For this review, take the finished solid that the model builds, in its own axes (mm). A direction names the side the tool comes from. Give positions to 0.01 mm unless a question says otherwise; leave off trailing zeros. Order: outer loops, then holes, each group sorted by start corner. A loop starts at its lowest first (then second) coordinate and runs counter-clockwise, first axis right, second up.
from build123d import *

# Parameters (mm, degrees)
AUFSATZ_LINEAR_AUSTRAGEN1_DEPTH = 3
AUFSATZ_LINEAR_AUSTRAGEN3_DEPTH = 3
AUFSATZ_LINEAR_AUSTRAGEN2_DEPTH = 20
AUFSATZ_LINEAR_AUSTRAGEN4_DEPTH = 8
FASE1_SIZE                      = 8
SCHNITT_LINEAR_AUSTRAGEN1_REACH = 119.702
SKIZZE5_R                       = 2.6
SCHNITT_LINEAR_AUSTRAGEN2_REACH = 178.395
SKIZZE6_R                       = 2.6
SCHNITT_LINEAR_AUSTRAGEN3_REACH = 178.395
SKIZZE7_R                       = 2.6
SCHNITT_LINEAR_AUSTRAGEN4_REACH = 140.701
SKIZZE8_R                       = 2.6


with BuildPart() as part:
    # Skizze1 → Aufsatz-Linear austragen1 (new body)
    with BuildSketch(Plane(origin=(0, 0, 0), x_dir=(1, 0, 0), z_dir=(0, 1, 0))):
        Polygon((-10, -84.737699009), (10, -84.737699009), (10, -64.737699009), (61.064491924, 23.708595467), (78.385, 33.708595467), (68.385, 51.029103542), (51.064491924, 41.029103542), (-51.064491924, 41.029103542), (-68.385, 51.029103542), (-78.385, 33.708595467), (-61.064491924, 23.708595467), (-10, -64.737699009), align=None)
    extrude(amount=AUFSATZ_LINEAR_AUSTRAGEN1_DEPTH)

    # Skizze3 → Aufsatz-Linear austragen3 (add)
    with BuildSketch(Plane.XZ):
        Polygon((0, -51.029103542), (-10, -41.029103542), (10, -41.029103542), align=None)
    extrude(amount=-AUFSATZ_LINEAR_AUSTRAGEN3_DEPTH)

    # Skizze2 → Aufsatz-Linear austragen2 (add)
    with BuildSketch(Plane.XZ):
        Polygon((-10.057735027, 64.637699009), (10.057735027, 64.637699009), (11.789785834, 61.637699009), (-11.789785834, 61.637699009), align=None)
        Polygon((61.006756897, -23.608595467), (50.94902187, -41.029103542), (47.484920255, -41.029103542), (59.27470609, -20.608595467), align=None)
        Polygon((-50.94902187, -41.029103542), (-61.006756897, -23.608595467), (-59.27470609, -20.608595467), (-47.484920255, -41.029103542), align=None)
    extrude(amount=AUFSATZ_LINEAR_AUSTRAGEN2_DEPTH)

    # Skizze4 → Aufsatz-Linear austragen4 (add)
    with BuildSketch(Plane.XZ):
        Polygon((-11.789785834, 61.637699009), (-16.408587988, 53.637699009), (-13.408587988, 53.637699009), (-8.789785834, 61.637699009), align=None)
        Polygon((11.789785834, 61.637699009), (8.789785834, 61.637699009), (13.408587988, 53.637699009), (16.408587988, 53.637699009), align=None)
        Polygon((59.27470609, -20.608595467), (54.655903936, -12.608595467), (53.155903936, -15.206671678), (57.77470609, -23.206671678), align=None)
        Polygon((47.484920255, -41.029103542), (48.984920255, -38.431027331), (39.747315948, -38.431027331), (38.247315948, -41.029103542), align=None)
        Polygon((-47.484920255, -41.029103542), (-38.247315948, -41.029103542), (-39.747315948, -38.431027331), (-48.984920255, -38.431027331), align=None)
        Polygon((-59.27470609, -20.608595467), (-57.77470609, -23.206671678), (-53.155903936, -15.206671678), (-54.655903936, -12.608595467), align=None)
    extrude(amount=AUFSATZ_LINEAR_AUSTRAGEN4_DEPTH)

    # Fase1
    # the kernel refuses this chamfer: 8 mm, written as the material it takes off along each edge
    with BuildSketch(Plane(origin=(-42.869171984, -8, -33.023814062), x_dir=(0.023812127644089447, 0.9996219169112968, 0.013747938305292782), z_dir=(-0.5000000000000003, 0, 0.8660254037844386))) as fase1_piece_1_section:
        Polygon((FASE1_SIZE * 0.999621916911, FASE1_SIZE * 0.0274958766106), (-FASE1_SIZE * 0.0274958766106, FASE1_SIZE * 0.999621916911), (0, 0), align=None)
    fase1_piece_1 = extrude(amount=44.146927807, mode=Mode.PRIVATE)
    fase1_piece_1 = split(fase1_piece_1, bisect_by=Plane(origin=(-56.186972779, 0, -15.224609283), z_dir=(0, -1, 0)), keep=Keep.TOP, mode=Mode.PRIVATE)
    add(fase1_piece_1, mode=Mode.SUBTRACT)
    with BuildSketch(Plane(origin=(-27.960583996, -8, -58.846245927), x_dir=(0.02381212764409005, 0.9996219169112968, 0.013747938305293118), z_dir=(-0.5, 0, 0.8660254037844387))) as fase1_piece_2_section:
        Polygon((FASE1_SIZE * 0.999621916911, FASE1_SIZE * 0.0274958766106), (-FASE1_SIZE * 0.0274958766106, FASE1_SIZE * 0.999621916911), (0, 0), align=None)
    fase1_piece_2 = extrude(amount=44.146927807, mode=Mode.PRIVATE)
    fase1_piece_2 = split(fase1_piece_2, bisect_by=Plane(origin=(-41.278384791, 0, -41.047041147), z_dir=(0, -1, 0)), keep=Keep.TOP, mode=Mode.PRIVATE)
    add(fase1_piece_2, mode=Mode.SUBTRACT)
    with BuildSketch(Plane(origin=(50.0340479, -8, -20.613884946), x_dir=(-0.023812127644090117, 0.9996219169112968, 0.013747938305293118), z_dir=(-0.49999999999999895, 0, -0.8660254037844393))) as fase1_piece_3_section:
        Polygon((FASE1_SIZE * 0.999621916911, FASE1_SIZE * 0.0274958766106), (-FASE1_SIZE * 0.0274958766106, FASE1_SIZE * 0.999621916911), (0, 0), align=None)
    fase1_piece_3 = extrude(amount=44.146927807, mode=Mode.PRIVATE)
    fase1_piece_3 = split(fase1_piece_3, bisect_by=Plane(origin=(41.278384791, 0, -41.047041147), z_dir=(0, -1, 0)), keep=Keep.TOP, mode=Mode.PRIVATE)
    add(fase1_piece_3, mode=Mode.SUBTRACT)
    with BuildSketch(Plane(origin=(64.942635888, -8, 5.208546918), x_dir=(-0.023812127644090537, 0.9996219169112968, 0.013747938305293455), z_dir=(-0.5000000000000016, 0, -0.8660254037844378))) as fase1_piece_4_section:
        Polygon((FASE1_SIZE * 0.999621916911, FASE1_SIZE * 0.0274958766106), (-FASE1_SIZE * 0.0274958766106, FASE1_SIZE * 0.999621916911), (0, 0), align=None)
    fase1_piece_4 = extrude(amount=44.146927807, mode=Mode.PRIVATE)
    fase1_piece_4 = split(fase1_piece_4, bisect_by=Plane(origin=(56.186972779, 0, -15.224609283), z_dir=(0, -1, 0)), keep=Keep.TOP, mode=Mode.PRIVATE)
    add(fase1_piece_4, mode=Mode.SUBTRACT)
    with BuildSketch(Plane(origin=(-7.164875916, -8, 53.637699009), x_dir=(0, -0.02749587661058627, 0.9996219169112968), z_dir=(1, 0, 0))) as fase1_piece_5_section:
        Polygon((FASE1_SIZE * 0.999621916911, -FASE1_SIZE * 0.0274958766106), (-FASE1_SIZE * 0.0274958766106, -FASE1_SIZE * 0.999621916911), (0, 0), align=None)
    fase1_piece_5 = extrude(amount=44.146927807, mode=Mode.PRIVATE)
    fase1_piece_5 = split(fase1_piece_5, bisect_by=Plane(origin=(14.908587988, 0, 61.735979971), z_dir=(0, -1, 0)), keep=Keep.TOP, mode=Mode.PRIVATE)
    add(fase1_piece_5, mode=Mode.SUBTRACT)
    with BuildSketch(Plane(origin=(-36.982051892, -8, 53.637699009), x_dir=(0, 0.9996219169112968, -0.027495876610586494), z_dir=(1, 0, 0))) as fase1_piece_6_section:
        Polygon((FASE1_SIZE * 0.999621916911, FASE1_SIZE * 0.0274958766106), (-FASE1_SIZE * 0.0274958766106, FASE1_SIZE * 0.999621916911), (0, 0), align=None)
    fase1_piece_6 = extrude(amount=44.146927807, mode=Mode.PRIVATE)
    fase1_piece_6 = split(fase1_piece_6, bisect_by=Plane(origin=(-14.908587988, 0, 56.27165043), z_dir=(0, -1, 0)), keep=Keep.TOP, mode=Mode.PRIVATE)
    add(fase1_piece_6, mode=Mode.SUBTRACT)

    # Skizze5 → Schnitt-Linear austragen1 (cut, up to next)
    with BuildSketch(Plane(origin=(0, 3, 0), x_dir=(1, 0, 0), z_dir=(0, 1, 0)), mode=Mode.PRIVATE) as schnitt_linear_austragen1_sk1:
        with Locations(Location((-64.724745962, 37.368849504, 0), (0, 0, 270))):
            Circle(SKIZZE5_R)
    schnitt_linear_austragen1_tool1 = extrude(schnitt_linear_austragen1_sk1.sketch, amount=-SCHNITT_LINEAR_AUSTRAGEN1_REACH, mode=Mode.PRIVATE) & part.part
    # Skizze5 → Schnitt-Linear austragen1 (cut, up to next)
    with BuildSketch(Plane(origin=(0, 3, 0), x_dir=(1, 0, 0), z_dir=(0, 1, 0)), mode=Mode.PRIVATE) as schnitt_linear_austragen1_sk2:
        with Locations(Location((64.724745962, 37.368849504, 0), (0, 0, 270))):
            Circle(SKIZZE5_R)
    schnitt_linear_austragen1_tool2 = extrude(schnitt_linear_austragen1_sk2.sketch, amount=-SCHNITT_LINEAR_AUSTRAGEN1_REACH, mode=Mode.PRIVATE) & part.part
    # Skizze5 → Schnitt-Linear austragen1 (cut, up to next)
    with BuildSketch(Plane(origin=(0, 3, 0), x_dir=(1, 0, 0), z_dir=(0, 1, 0)), mode=Mode.PRIVATE) as schnitt_linear_austragen1_sk3:
        with Locations(Location((-0.028867513, -74.687699009, 0), (0, 0, 270))):
            Circle(SKIZZE5_R)
    schnitt_linear_austragen1_tool3 = extrude(schnitt_linear_austragen1_sk3.sketch, amount=-SCHNITT_LINEAR_AUSTRAGEN1_REACH, mode=Mode.PRIVATE) & part.part
    add(schnitt_linear_austragen1_tool1.solids().sort_by_distance((-64.724746, 3, -37.36885))[0], mode=Mode.SUBTRACT)
    add(schnitt_linear_austragen1_tool2.solids().sort_by_distance((64.724746, 3, -37.36885))[0], mode=Mode.SUBTRACT)
    add(schnitt_linear_austragen1_tool3.solids().sort_by_distance((-0.028868, 3, 74.687699))[0], mode=Mode.SUBTRACT)

    # Skizze6 → Schnitt-Linear austragen2 (cut, up to next)
    with BuildSketch(Plane(origin=(53.379813173, 0, -30.818849504), x_dir=(0.49999999999999967, 0, 0.8660254037844389), z_dir=(-0.8660254037844389, 0, 0.49999999999999967)), mode=Mode.PRIVATE) as schnitt_linear_austragen2_sk1:
        with Locations((0, -10)):
            Circle(SKIZZE6_R)
    schnitt_linear_austragen2_tool1 = extrude(schnitt_linear_austragen2_sk1.sketch, amount=-SCHNITT_LINEAR_AUSTRAGEN2_REACH, mode=Mode.PRIVATE) & part.part
    add(schnitt_linear_austragen2_tool1.solids().sort_by_distance((53.379813, -10, -30.81885))[0], mode=Mode.SUBTRACT)

    # Skizze7 → Schnitt-Linear austragen3 (cut, up to next)
    with BuildSketch(Plane(origin=(-53.379813173, 0, -30.818849504), x_dir=(0.5000000000000007, 0, -0.8660254037844383), z_dir=(0.8660254037844383, 0, 0.5000000000000007)), mode=Mode.PRIVATE) as schnitt_linear_austragen3_sk1:
        with Locations((0, -10)):
            Circle(SKIZZE7_R)
    schnitt_linear_austragen3_tool1 = extrude(schnitt_linear_austragen3_sk1.sketch, amount=-SCHNITT_LINEAR_AUSTRAGEN3_REACH, mode=Mode.PRIVATE) & part.part
    add(schnitt_linear_austragen3_tool1.solids().sort_by_distance((-53.379813, -10, -30.81885))[0], mode=Mode.SUBTRACT)

    # Skizze8 → Schnitt-Linear austragen4 (cut, up to next)
    with BuildSketch(Plane(origin=(0, 0, 61.637699009), x_dir=(-1, 0, 0), z_dir=(0, 0, -1)), mode=Mode.PRIVATE) as schnitt_linear_austragen4_sk1:
        with Locations((0, -10)):
            Circle(SKIZZE8_R)
    schnitt_linear_austragen4_tool1 = extrude(schnitt_linear_austragen4_sk1.sketch, amount=-SCHNITT_LINEAR_AUSTRAGEN4_REACH, mode=Mode.PRIVATE) & part.part
    add(schnitt_linear_austragen4_tool1.solids().sort_by_distance((0, -10, 61.637699))[0], mode=Mode.SUBTRACT)


solid = part.part
1) We need section D-D on x = -33. Give the boundary of the cut face in (y, z), then the cut area to 3 significant figures.
Answer sheet:
outline: (0, -41.03) - (3, -41.03) - (3, 24.9) - (0, 24.9) - close
area: 198 mm2
2) Draft analysis for pull direction Z (two halves, no side actions). For faces 6 (the face through (-1, 3, 1)), 7 (the face through (-43.541, -3.944, -39.748)), 8 (the face through (62.187, 1.521, -37.932)), 9 (the face through (54.379, -12.538, -32.046)), state which applies: +Z half, -Z half, draft (parallel to the pull), parting line (faces both ways), or undercut.
Answer sheet:
face 6: draft
face 7: +Z half
face 8: undercut
face 9: undercut
3) We need section C-C on z = 68. Give the boundary of the cut face in (x, y).
Answer sheet:
outline: (-10, 0) - (10, 0) - (10, 3) - (-10, 3) - close
4) Tool access review of faces 1 (the face through (-40, -1, -41.029)), 2 (the face through (68, 0, -38)), 3 (the face through (56.19, -3.94, -17.83)), 4 (the face through (3, -10, 61.638)), 5 (the face through (73.455, 1.479, -42.248)): name each direction out of +Z, -Z, +X, -X, +Y, -Y from which nothing blocks a thin tool from reaching the whole face with its end or side.
Answer sheet:
face 1: -Z, +Y, -Y
face 2: -Z, +X, -Y
face 3: +Z, -Y
face 4: -Z, -Y
face 5: -Z, +X, +Y, -Y
5) We need section B-B on y = -10. Give the boundary of the cut face in (x, z).
Answer sheet:
outline: (-61.01, -23.61) - (-57.28, -30.07) - (-54.68, -28.57) - (-59.27, -20.61) - close; (-54.68, -34.57) - (-50.95, -41.03) - (-47.48, -41.03) - (-52.08, -33.07) - close; (-11.79, 61.64) - (-2.6, 61.64) - (-2.6, 64.64) - (-10.06, 64.64) - close; (2.6, 61.64) - (11.79, 61.64) - (10.06, 64.64) - (2.6, 64.64) - close; (47.48, -41.03) - (50.95, -41.03) - (54.68, -34.57) - (52.08, -33.07) - close; (54.68, -28.57) - (57.28, -30.07) - (61.01, -23.61) - (59.27, -20.61) - close
6) To check wall thickness, follow line 1 (Y direction, x = 0, z = 62.4); line 2 (Z direction, x = 1, y = -2); line 3 (Y direction, x = -57.5, z = -41). State the ranges of each line that lie inside material, in increasing order.
Answer sheet:
line 1: y = -20 to -12.6, -7.4 to 3
line 2: z = 61.64 to 64.64
line 3: y = 0 to 3
7) Clearance check with flat-ended pins moving along their axes: pin 1 (6 mm diameter, centred on x = -1, y = -12, fed in from -Z); pin 2 (8.5 mm diameter, centred on x = -0.03, z = 74.69, fed in from -Y); pin 3 (6 mm diameter, centred on x = 1, y = -6.5, fed in from +Z). State where each tip first meets the part, or that it passes through.
Answer sheet:
pin 1: stops at z = 61.64
pin 2: stops at y = 0
pin 3: stops at z = 64.64
8) We need section A-A on y = -2.25. Give the boundary of the cut face in (x, z), then the cut area to 3 significant figures.
Answer sheet:
outline: (-61.01, -23.61) - (-50.95, -41.03) - (-40.85, -41.03) - (-42.35, -38.43) - (-48.98, -38.43) - (-57.77, -23.21) - (-54.45, -17.46) - (-55.95, -14.86) - close; (-15.11, 55.89) - (-12.11, 55.89) - (-8.79, 61.64) - (8.79, 61.64) - (12.11, 55.89) - (15.11, 55.89) - (10.06, 64.64) - (-10.06, 64.64) - close; (40.85, -41.03) - (50.95, -41.03) - (61.01, -23.61) - (55.95, -14.86) - (54.45, -17.46) - (57.77, -23.21) - (48.98, -38.43) - (42.35, -38.43) - close
area: 300 mm2
